Geometry check sheet. Reference: drawing and pictorial views, mm from the part's lowest x, y, z. A direction names the side the tool comes from. Round coordinates to 2 decimals unless told otherwise and drop trailing zeros. Loops run counter-clockwise (first coordinate to the right, second up) from the corner with the lowest first, then second, coordinate; pieces in that order, holes last. Notation, with made-up numbers: (23, 5) - (79, 5) arc R34 ccw to (79, 36) - close; hole circle Ø7 at (53, 37). An arc over 180 degrees is marked (long way). Return JSON: item names as keys, results as strings.
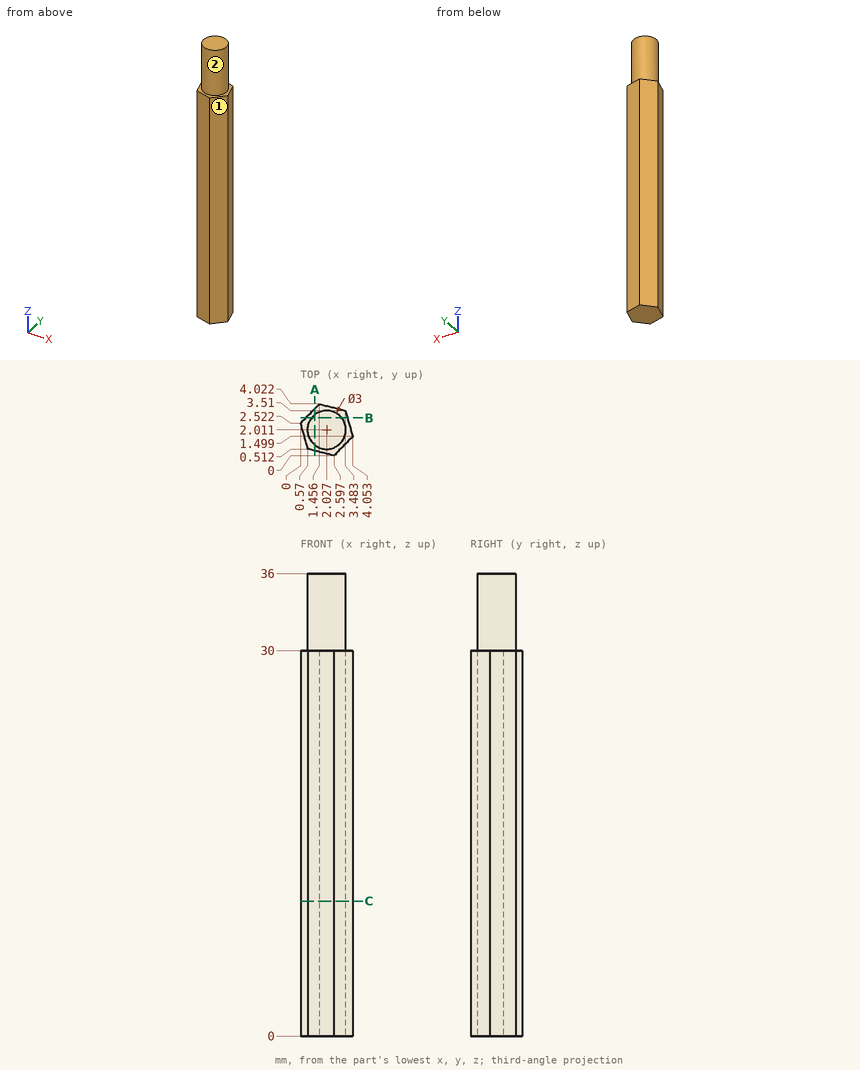
Q1. Sectioned sample at B-B (y = 2.95). Enter the section's corners in (x, z) (1 decimal).
Answer key:
{"outline": "(0.4, 0) - (3.6, 0) - (3.6, 30) - (3.2, 30) - (3.2, 36) - (0.9, 36) - (0.9, 30) - (0.4, 30) - close"}
Q2. Sectioned sample at C-C (z = 10.5). Enter the section's corners in (x, y).
Answer key:
{"outline": "(0, 2.52) - (0.57, 0.51) - (2.6, 0) - (4.05, 1.5) - (3.48, 3.51) - (1.46, 4.02) - close"}
Q3. Sectioned sample at A-A (x = 1.1). Enter the section's corners in (y, z) (1 decimal).
Answer key:
{"outline": "(0.4, 0) - (3.7, 0) - (3.7, 30) - (3.2, 30) - (3.2, 36) - (0.8, 36) - (0.8, 30) - (0.4, 30) - close"}
Q4. Scan lines: probe 1 along Z at (x, y) = (3.8, 2.2); probe 2 along X at (y, z) = (2.9, 18.5) (1 decimal); probe 3 along X at (y, z) = (1.6, 6.5) (1 decimal). Record each from-to range of solid material in increasing order. Write a range as [from, to].
Answer key:
{"probe 1": "z = [0, 30]", "probe 2": "x = [0.4, 3.7]", "probe 3": "x = [0.3, 4]"}
Q5. Tool access check on the marked faces 1 and 2. Record the directions out of +Z, -Z, +X, -X, +Y, -Y that give a thin tool (end or side, any length) a straight path to the whole face; none if there is none.
Answer key:
{"face 1": "+Z, -Z, +X, -Y", "face 2": "+Z"}
Q6. Depth check by flat-ended pin: P1, Ø1.5, axis at y = 3, z = 14, coming from the -X side. Enter the tip coordinate at first touch or a pass-through.
Answer key:
{"P1": "stops at x = 0"}
